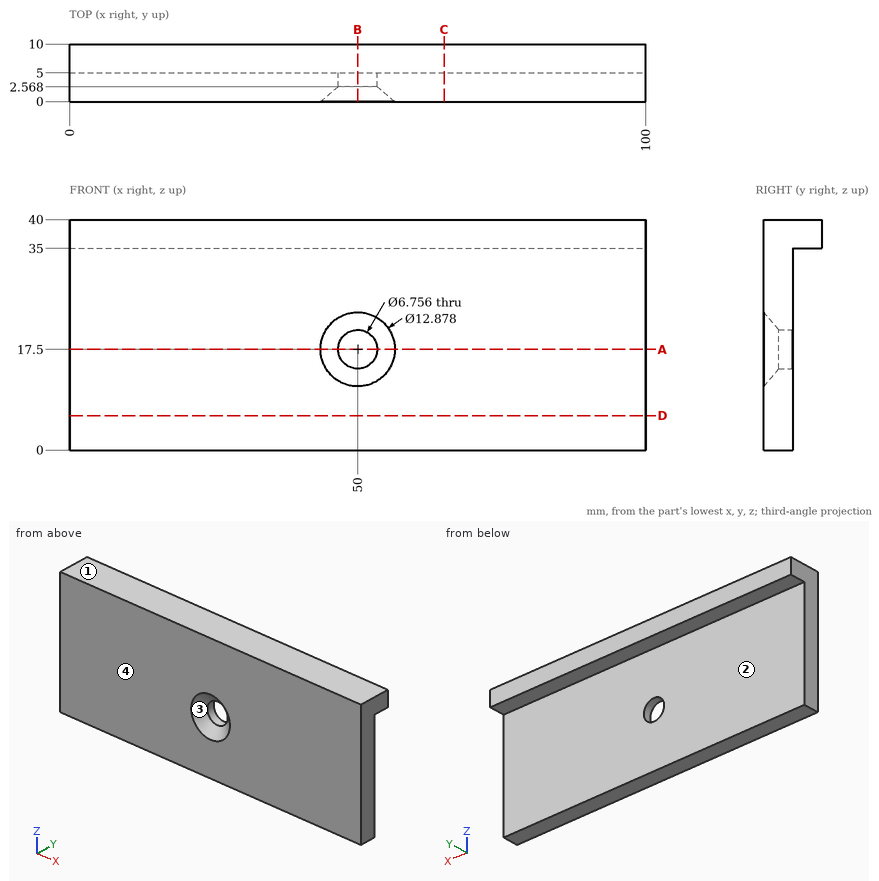
Answer from the drawing. Dimensions are ordinates in mm from the lowest x, y and z of the part. A direction names the side the tool comes from. Round coordinates to 2 decimals unless told otherwise and drop trailing zeros. Loops run counter-clockwise (first coordinate to the right, second up) from the corner with the lowest first, then second, coordinate; pieces in that order, holes last.
Q1. Section A-A on z = 17.5 is taken. Write down the section's boundary in (x, y).
Q2. Each of these flat-tipped pins is pushed along its axis until it touches: pin 1 (17.5 mm diameter, centred on x = 53, z = 25, fed in from +Y); pin 2 (2.5 mm diameter, centred on x = 64, y = 7.5, fed in from -Z). Where does it stop, or does it pass through?
Q3. Consider probe 1 along Z at (x, y) = (50, 3.2); probe 2 along X at (y, z) = (4.35, 17.5); probe 3 along Y at (x, z) = (21.5, 8.5). Determine where each line is inside the solid, lowest interval first.
Q4. Section B-B on x = 50 is taken. Write down the section's boundary in (y, z), and give its area (3 significant figures).
Q5. Section C-C on x = 65 is taken. Write down the section's boundary in (y, z).
Q6. Determine the mould class of the marked faces 3 and 4 for opening direction X: released by +X, released by -X, zero draft, split by the parting line, or undercut.
Q7. Section D-D on z = 6 is taken. Write down the section's boundary in (x, y).
Q8. Which of the six approach directions +Z, -Z, +X, -X, +Y, -Y give full straight-line access (tool end or side, diameter ignored) to the marked faces 1 and 2?
Output:
1. outline: (0, 0) - (43.56, 0) - (46.62, 2.57) - (46.62, 5) - (0, 5) - close; (53.38, 2.57) - (56.44, 0) - (100, 0) - (100, 5) - (53.38, 5) - close
2. pin 1: stops at y = 5
2. pin 2: stops at z = 35
3. probe 1: z = 0 to 14.12, 20.88 to 40
3. probe 2: x = 0 to 46.62, 53.38 to 100
3. probe 3: y = 0 to 5
4. outline: (0, 0) - (5, 0) - (5, 14.12) - (2.57, 14.12) - (0, 11.06) - close; (0, 23.94) - (2.57, 20.88) - (5, 20.88) - (5, 35) - (10, 35) - (10, 40) - (0, 40) - close
4. area: 183 mm2
5. outline: (0, 0) - (5, 0) - (5, 35) - (10, 35) - (10, 40) - (0, 40) - close
6. face 3: undercut
6. face 4: zero draft
7. outline: (0, 0) - (100, 0) - (100, 5) - (0, 5) - close
8. face 1: +Z, +X, -X, +Y, -Y
8. face 2: -Z, +X, -X, +Y
